Autodesk Inventor part; units mm, degrees
ref_plane "YZ Plane" through (0, 0, 0) normal (1, 0, 0) x (0, 1, 0)
ref_plane "XZ Plane" through (0, 0, 0) normal (0, 1, 0) x (-1, 0, 0)
ref_plane "XY Plane" through (0, 0, 0) normal (0, 0, 1) x (1, 0, 0)
sketch "Skizze1" plane through (0, 0, 0) normal (0, 1, 0) x (-1, 0, 0)
  line L0 (0, 0) -> (180, 0)
  line L1 (180, -100) -> (0, -100)
  line L2 (0, -100) -> (0, 0)
  line L3 (5, -95) -> (5, -5)
  line L4 (5, -5) -> (170, -5)
  line L5 (5, -95) -> (170, -95)
  line L6 (170, -95) -> (170, -97.5)
  line L7 (170, -97.5) -> (180, -97.5)
  line L8 (170, -5) -> (170, -2.5)
  line L9 (170, -2.5) -> (180, -2.5)
  line L10 (180, 0) -> (180, -2.5)
  line L11 (180, -100) -> (180, -97.5)
  dimension "d0" = 180
  dimension "d1" = 100
  dimension "d2" = 90
  dimension "d3" = 165
extrude "Extrusion1" add sketch "Skizze1" along normal blind 25
sketch "Skizze2" plane through (-5, 0, -95) normal (-1, 0, 0) x (0, 0, 1)
  line L0 (90, 0) -> (90, 25)
  line L1 (0, 0) -> (90, 0)
  line L2 (90, 0) -> (90, 25)
  line L3 (0, 25) -> (90, 25)
  line L4 (0, 0) -> (0, 25)
  line L5 (0, 0) -> (90, 0)
  line L6 (90, 0) -> (90, 2.5)
  line L7 (90, 2.5) -> (0, 2.5)
  line L8 (0, 2.5) -> (0, 0)
  point P0 (95, 0)
  dimension "d6" = 90
  dimension "d7" = 2.5
extrude "Extrusion2" add sketch "Skizze2" along normal blind 165 contours L1 L4 L7 L0
properties part number "Schublade Teil B"
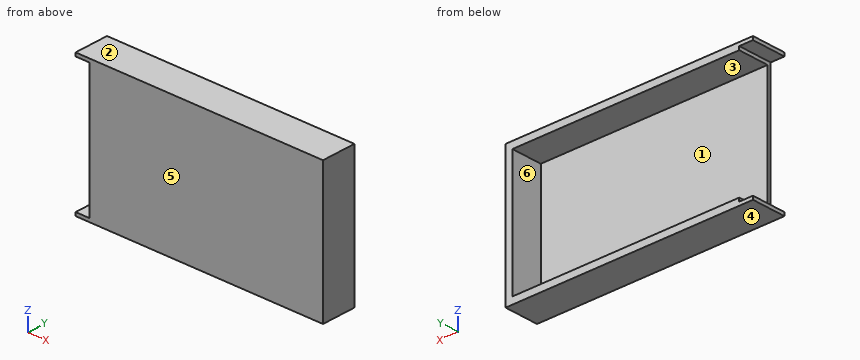
Read the model definition and answer for the solid it produces. Units are mm, in the model's axes. Face numbers are marked on the shaded views. A direction names the side the tool comes from. Coordinates: 2 decimals unless noted, no trailing zeros. Loops run counter-clockwise (first coordinate to the right, second up) from the corner with the lowest first, then second, coordinate; pieces in that order, holes last.
Q1. This flat-tipped pin is pushed along its axis until it touches: pin 1 Ø4 at (y, z) = (11.5, -44.5) entering from -X. Where does it stop, or does it pass through?
Q2. Consider probe 1 along Z at (x, y) = (-37, 21.75); probe 2 along Z at (x, y) = (-171.5, 5.25); probe 3 along Y at (x, z) = (-160.5, -94). Determine where each line is inside the solid, lowest interval first.
Q3. The part is cut by section C-C on z = -34.5. Write down the section's boundary in (x, y), and give its area (4 significant figures).
Q4. The part is cut by section A-A on y = 22.75. Write down the section's boundary in (x, z).
Q5. The part is cut by section B-B on x = -90. Write down the section's boundary in (y, z).
Q6. Which of the six approach directions +Z, -Z, +X, -X, +Y, -Y give full straight-line access (tool end or side, diameter ignored) to the marked faces 1 and 2?
Q7. The mould has two halves that part along Z. Classify the marked faces 3, 4, 5 and 6: +Z half, -Z half, draft (parallel to the pull), parting line (faces both ways), or undercut.
Results below:
1. pin 1: stops at x = -5
2. probe 1: z = -100 to -95, -5 to 0
2. probe 2: z = -100 to -97.5, -2.5 to 0
2. probe 3: y = 0 to 2.5
3. outline: (-170, 0) - (0, 0) - (0, 25) - (-5, 25) - (-5, 2.5) - (-170, 2.5) - close
3. area: 537.5 mm2
4. outline: (-180, -100) - (0, -100) - (0, 0) - (-180, 0) - (-180, -2.5) - (-170, -2.5) - (-170, -5) - (-5, -5) - (-5, -95) - (-170, -95) - (-170, -97.5) - (-180, -97.5) - close
5. outline: (0, -100) - (25, -100) - (25, -95) - (2.5, -95) - (2.5, -5) - (25, -5) - (25, 0) - (0, 0) - close
6. face 1: -X, +Y
6. face 2: +Z, +X, -X, +Y, -Y
7. face 3: undercut
7. face 4: -Z half
7. face 5: draft
7. face 6: undercut
